Design review of the part shown in the three views and the two pictorial views. Dimensions are in mm from the part's minimum x, y and z. A direction names the side the tool comes from. Give positions to 0.01 mm unless a question says otherwise; leave off trailing zeros. Order: outer loops, then holes, each group sorted by start corner. A loop starts at its lowest first (then second) coordinate and runs counter-clockwise, first axis right, second up.
Item 1: Consider section C-C (x = 36.83). Give the boundary of the cut face in (y, z).
Item 2: For P1, Ø3.5, axis at x = 36.83, y = 69.85, coming from the +Z side; P2, Ø9.5, axis at y = 36, z = 18, coming from the -X side; P3, Ø4, axis at x = 24, z = 18, coming from the -Y side; P4, Ø6, axis at x = 7.5, y = 26, coming from the +Z side, all flat-tipped, find the tip position at first contact; note any pin that passes through.
Item 3: Consider section B-B (y = 15.24). Give the boundary of the cut face in (x, z) (1 decimal), plus the area to 3 significant figures.
Item 4: Consider section A-A (z = 18.75). Give the boundary of the cut face in (x, y).
Item 5: Consider section D-D (x = 24.13). Give the boundary of the cut face in (y, z), plus the area to 3 significant figures.
Item 6: For probe 1 along X at (y, z) = (7.62, 2.5); probe 2 along Y at (x, z) = (36.83, 7.25); probe 3 along X at (y, z) = (47, 12.5), list the stretches that pass through material, from the lowest coordinate up.
Item 7: Machinability: for the marked faces 1, 2 and 3, which of the approach directions +Z, -Z, +X, -X, +Y, -Y give a long, thin tool a straight path to every point of the face, cutting with its end or side? Answer none if there is none.
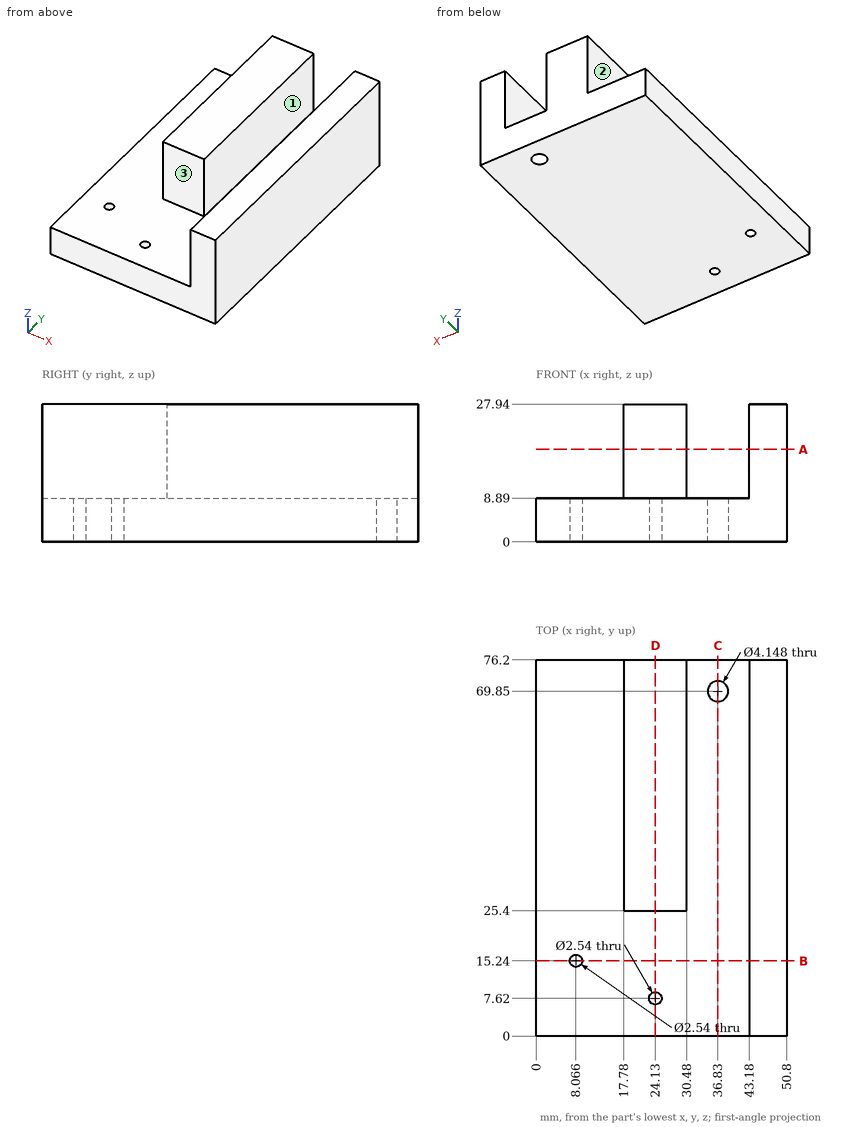
Resolved:
1. outline: (0, 0) - (67.78, 0) - (67.78, 8.89) - (0, 8.89) - close; (71.92, 0) - (76.2, 0) - (76.2, 8.89) - (71.92, 8.89) - close
2. P1: passes through
2. P2: stops at x = 17.78
2. P3: stops at y = 25.4
2. P4: stops at z = 8.89
3. outline: (0, 0) - (6.8, 0) - (6.8, 8.9) - (0, 8.9) - close; (9.3, 0) - (50.8, 0) - (50.8, 27.9) - (43.2, 27.9) - (43.2, 8.9) - (9.3, 8.9) - close
3. area: 574 mm2
4. outline: (17.78, 25.4) - (30.48, 25.4) - (30.48, 76.2) - (17.78, 76.2) - close; (43.18, 0) - (50.8, 0) - (50.8, 76.2) - (43.18, 76.2) - close
5. outline: (0, 0) - (6.35, 0) - (6.35, 8.89) - (0, 8.89) - close; (8.89, 0) - (76.2, 0) - (76.2, 27.94) - (25.4, 27.94) - (25.4, 8.89) - (8.89, 8.89) - close
5. area: 1,620 mm2
6. probe 1: x = 0 to 22.86, 25.4 to 50.8
6. probe 2: y = 0 to 67.78, 71.92 to 76.2
6. probe 3: x = 17.78 to 30.48, 43.18 to 50.8
7. face 1: +Z, +Y, -Y
7. face 2: +Z, -X, +Y, -Y
7. face 3: +Z, -X, -Y
